from build123d import *

# Parameters (mm, degrees)
F0_W     = 6.35
F0_H     = 34.29
F1_DEPTH = 6.35
F2_R     = 3.17499
F3_R     = 1.651
F4_DEPTH = 6.35


# Not quite as in the source:
# - a fillet or chamfer is up to 0.001 mm smaller than in the source, because OpenCascade refuses the exact size


with BuildPart() as f1:
    # F0 (on Top) → F1 (new body)
    with BuildSketch(Plane.XY):
        Rectangle(F0_W, F0_H)
    extrude(amount=F1_DEPTH)

    # F2 (radius 3.175 in the source; OpenCascade refuses exactly that, so slightly less here)
    f2_edges = [f1.edges().sort_by_distance(p)[0] for p in [
        (3.175, 17.145, 3.175),
        (-3.175, 17.145, 3.175),
        (3.175, -17.145, 3.175),
        (-3.175, -17.145, 3.175),
    ]]
    fillet(f2_edges, radius=F2_R)

    # F3 (on face) → F4 (cut, through all)
    with BuildSketch(Plane.XY.offset(6.35)):
        with Locations((0, -13.97)):
            Circle(F3_R)
        with Locations((0, 13.97)):
            Circle(F3_R)
    extrude(amount=-F4_DEPTH, mode=Mode.SUBTRACT)


solid = f1.part
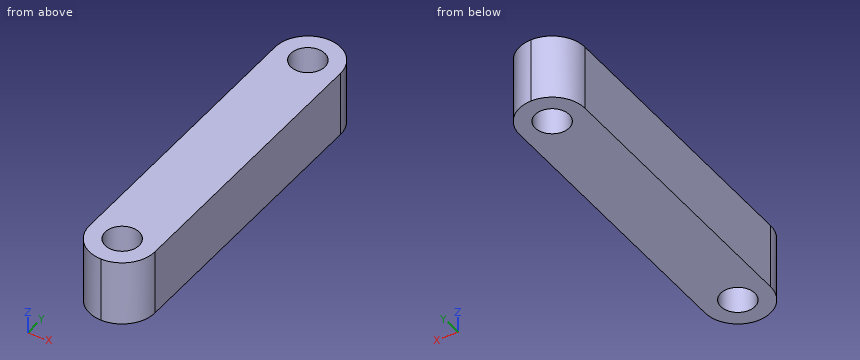
Model file for the job. Use its own axes, mm. Coordinates: 2 decimals unless noted, no trailing zeros. Order: outer loops, then holes, each group sorted by start corner. A loop starts at its lowest first (then second) coordinate and runs counter-clockwise, first axis right, second up. Notation, with made-up numbers: (-36.75, 23) -> (1.25, 23) arc R31 ccw to (1.25, 48) -> close; hole circle Ø3 at (56, 17.25). An arc over 180 degrees is marked (long way). Return JSON: item names as keys, results as strings. Group by question number.
Item 1: Saw through at A-A on z = 5.75. State how many separate pieces and enclosed holes the cut face has, then the cut area to 3 significant figures.
Item 2: Saw through at B-B on x = 0.75. Write the cut outline in (y, z), then the cut area to 3 significant figures.
Item 3: Saw through at C-C on x = -2.5. Write the cut outline in (y, z), then the cut area to 3 significant figures.
Item 4: Wall check: line 1 along Y through (x, z) = (0, 4.75) (3 decimals); line 2 along Y through (x, z) = (0.5, 2.25); line 3 along X through (y, z) = (14.5, 2.5). Give the ranges that are in metal, low to high. Write a range as [from, to].
Item 5: Flat gauge pins, fed straight in: P1, Ø1.5, axis at x = -2, y = 10, coming from the -Z side; P2, Ø1.5, axis at x = 1.5, z = 2, coming from the +Y side; P3, Ø1, axis at x = 2, z = 3.5, coming from the -Y side. Where does each tip first touch, or does it go through?
Values found:
{
 "1": {"separate pieces": "1", "enclosed holes": "2", "area": "192 mm2"},
 "2": {"outline": "(-17.06, 0) -> (-15.44, 0) -> (-15.44, 6.35) -> (-17.06, 6.35) -> close; (-12.5, 0) -> (12.5, 0) -> (12.5, 6.35) -> (-12.5, 6.35) -> close; (15.44, 0) -> (17.06, 0) -> (17.06, 6.35) -> (15.44, 6.35) -> close", "area": "179 mm2"},
 "3": {"outline": "(-15.93, 0) -> (15.93, 0) -> (15.93, 6.35) -> (-15.93, 6.35) -> close", "area": "202 mm2"},
 "4": {"line 1": "y = [-17.145, -15.621], [-12.319, 12.319], [15.621, 17.145]", "line 2": "y = [-17.11, -15.54], [-12.4, 12.4], [15.54, 17.11]", "line 3": "x = [-3.13, -1.56], [1.56, 3.13]"},
 "5": {"P1": "stops at z = 0", "P2": "stops at y = 17.06", "P3": "stops at y = -16.77"}
}
